```python
from build123d import *

# Parameters (mm, degrees)
SKETCH1_W             = 5.3
SKETCH1_H             = 2.6
BOSS_EXTRUDE1_DEPTH   = 6.2
BOSS_EXTRUDE1_2_DEPTH = 6.2
SKETCH2_W             = 5.3
SKETCH2_H             = 8.7
BOSS_EXTRUDE2_DEPTH   = 2
SKETCH3_W             = 1
SKETCH3_H             = 4.1
CUT_EXTRUDE1_DEPTH    = 2
SKETCH4_R             = 0.25
BOSS_EXTRUDE3_DEPTH   = 6


with BuildPart() as part:
    # Sketch1 → Boss-Extrude1 (new body)
    with BuildSketch(Plane.XY):
        with Locations((0, 3.05)):
            Rectangle(SKETCH1_W, SKETCH1_H)
    extrude(amount=BOSS_EXTRUDE1_DEPTH)



with BuildPart() as body_2:
    # Sketch1 → Boss-Extrude1 2 (new body)
    with BuildSketch(Plane.XY):
        with Locations((0, -3.05)):
            Rectangle(SKETCH1_W, SKETCH1_H)
    extrude(amount=BOSS_EXTRUDE1_2_DEPTH)


with BuildPart() as part_1:
    add(part.part)

    add(body_2.part)  # Boss-Extrude2 merges body 2
    # Sketch2 → Boss-Extrude2 (add)
    with BuildSketch(Plane(origin=(0, 0, 0), x_dir=(-1, 0, 0), z_dir=(0, 0, -1))):
        Rectangle(SKETCH2_W, SKETCH2_H)
    extrude(amount=BOSS_EXTRUDE2_DEPTH)

    # Sketch3 → Cut-Extrude1 (cut)
    with BuildSketch(Plane.XY.offset(6.2)):
        Rectangle(SKETCH3_W, SKETCH3_H)
    extrude(amount=-CUT_EXTRUDE1_DEPTH, mode=Mode.SUBTRACT)

    # Sketch4 → Boss-Extrude3 (add)
    with BuildSketch(Plane(origin=(0, 0, -2), x_dir=(-1, 0, 0), z_dir=(0, 0, -1))):
        with Locations((-1, -3.225)):
            Circle(SKETCH4_R)
        with Locations(Location((1, -3.225, 0), (0, 0, 180))):
            Circle(SKETCH4_R)
        with Locations((1, 3.225)):
            Circle(SKETCH4_R)
        with Locations(Location((-1, 3.225, 0), (0, 0, 180))):
            Circle(SKETCH4_R)
    extrude(amount=BOSS_EXTRUDE3_DEPTH)


solid = part_1.part
```
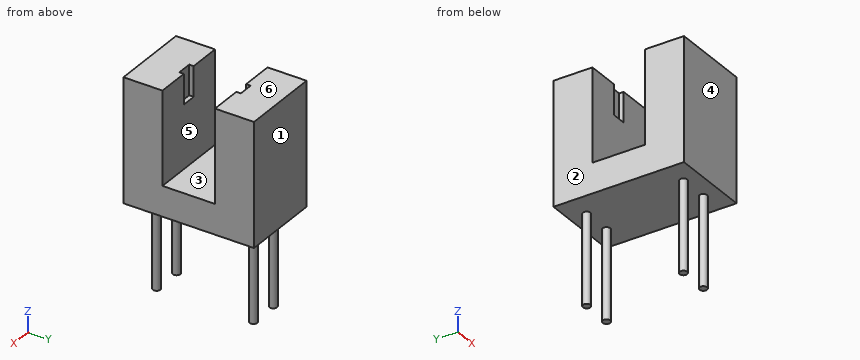
Input: part model. Units: mm. Frame: model coordinates. Face numbers are marked on the shaded views. A direction names the side the tool comes from. Coordinates: 2 decimals unless noted, no trailing zeros. Write each loop counter-clockwise with the first axis right and the second up, starting at its lowest first coordinate (ties: lowest second). Pieces come first, ordered by that corner, then holes. Notation, with made-up numbers: (0.25, 46) - (54.25, 46) arc R15 cw to (54.25, 69) - close; hole circle Ø8 at (-35, 43.25). An arc over 180 degrees is marked (long way). Put each result on its own line as item: value. Start each with the question number.
1) Ray query, L1, parallel to Y at x = 1.3, z = 3; L2, parallel to Z at x = -2.4, y = 1; L3, parallel to Y at x = 0.1, z = 4.75. Return the intervals inside material, ascending.
2) Cut plane D-D (z = -6.5). Return the cut outline in (x, y) (3 decimals), plus the area to 3 significant figures.
3) Contact query for flat-ended pins moving along their axis: pin 1 (1 mm diameter, centred on x = 0, y = 0.5, fed in from +Z); pin 2 (1.5 mm diameter, centred on x = 1, z = -5.5, fed in from -Y) (3 decimals). Output: stop coordinate, or through.
4) Cut plane A-A (z = 1). Return the cut outline in (x, y).
5) Cut plane B-B (x = 0.05). Return the cut outline in (y, z), plus the area to 3 significant figures.
6) Reachability of the marked faces 5 and 6 from +Z, -Z, +X, -X, +Y, -Y: full face, straight path, thin tool, end or side. Return the list, or none.
7) Cut plane C-C (y = 0.25). Return the cut outline in (x, z).
8) Mould query, pull axis Y, two halves, no side actions, for the marked faces 1, 2, 3 and 4. Classes: pulls with the +Y half, pulls with the -Y half, needs draft (parallel to the pull), parting line crosses it, or undercut.
Resolved:
1. L1: y = -4.35 to -1.75, 1.75 to 4.35
1. L2: z = -2 to 0
1. L3: y = -4.35 to -2.05, 2.05 to 4.35
2. outline: circle Ø0.5 at (-1, -3.225); circle Ø0.5 at (-1, 3.225); circle Ø0.5 at (1, -3.225); circle Ø0.5 at (1, 3.225)
2. area: 0.785 mm2
3. pin 1: stops at z = 0
3. pin 2: stops at y = -3.475
4. outline: (-2.65, -4.35) - (2.65, -4.35) - (2.65, -1.75) - (-2.65, -1.75) - close; (-2.65, 1.75) - (2.65, 1.75) - (2.65, 4.35) - (-2.65, 4.35) - close
5. outline: (-4.35, -2) - (4.35, -2) - (4.35, 6.2) - (2.05, 6.2) - (2.05, 4.2) - (1.75, 4.2) - (1.75, 0) - (-1.75, 0) - (-1.75, 4.2) - (-2.05, 4.2) - (-2.05, 6.2) - (-4.35, 6.2) - close
5. area: 48.4 mm2
6. face 5: +Z, +X, -X
6. face 6: +Z, +X, -X, +Y, -Y
7. outline: (-2.65, -2) - (2.65, -2) - (2.65, 0) - (-2.65, 0) - close
8. face 1: pulls with the +Y half
8. face 2: needs draft
8. face 3: undercut
8. face 4: pulls with the -Y half
